The listing builds one solid part. Answer for the finished solid, in the listing's coordinates (mm). Coordinates: 2 decimals unless noted, no trailing zeros. Order: outer loops, then holes, each group sorted by start corner. A loop starts at its lowest first (then second) coordinate and runs counter-clockwise, first axis right, second up. Notation, with made-up numbers: (-34.75, 11.25) - (-27.75, 11.25) arc R7 ccw to (-27.75, 23.25) - close; hole circle Ø4 at (-7.5, -21.75). An arc over 180 degrees is marked (long way). Use one line per item in the form item = value. Start each with the question number.
Item 1: Section B-B, the plane x = -55 is taken. Write down the section's boundary in (y, z) (3 decimals).
Item 2: Consider line 1 along X through (y, z) = (2, -5); line 2 along X through (y, z) = (1.15, -7.5); line 3 along Z through (x, y) = (-3.5, 2.75). Determine where each line is inside the solid, lowest interval first. Write a range as [from, to].
Item 3: Section C-C, the plane y = 2.6 is taken. Write down the section's boundary in (x, z), and give its area (3 significant figures).
Item 4: Each of these flat-tipped pins is pushed along its axis until it touches: pin 1 Ø6.5 at (x, z) = (-5, -5) entering from +Y (3 decimals); pin 2 Ø2.5 at (x, z) = (-55, -17.82) entering from -Y. Where does it stop, or does it pass through?
Item 5: Section A-A, the plane z = -5 is taken. Write down the section's boundary in (x, y) (3 decimals).
from build123d import *

# Parameters (mm, degrees)
SKETCH1_W                 = 60
SKETCH1_H                 = 25
BOSS_EXTRUDE1_DEPTH       = 3.175
M5_CLEARANCE_HOLE2_D      = 5.5
M5_CLEARANCE_HOLE2_DEPTH  = 15
M5_CLEARANCE_HOLE2_TIP    = 1.652366702
M5X0_8_TAPPED_HOLE2_D     = 4.2
M5X0_8_TAPPED_HOLE2_DEPTH = 15
M5X0_8_TAPPED_HOLE2_TIP   = 1.2618073


with BuildPart() as part:
    # Sketch1 → Boss-Extrude1 (new body)
    with BuildSketch(Plane(origin=(0, 0, 0), x_dir=(1, 0, 0), z_dir=(0, 1, 0))):
        with Locations((-30, 12.5)):
            Rectangle(SKETCH1_W, SKETCH1_H)
    extrude(amount=BOSS_EXTRUDE1_DEPTH)

    # M5 Clearance Hole2
    with Locations(Plane(origin=(-55, 3.175, -5), x_dir=(0, 0, 1), z_dir=(0, 1, 0))):
        with Locations((0, 0), (0, 50)):
            Hole(M5_CLEARANCE_HOLE2_D / 2, depth=M5_CLEARANCE_HOLE2_DEPTH)
            with Locations((0, 0, -(M5_CLEARANCE_HOLE2_DEPTH + M5_CLEARANCE_HOLE2_TIP / 2))):  # 118° drill point
                Cone(0, M5_CLEARANCE_HOLE2_D / 2, M5_CLEARANCE_HOLE2_TIP, mode=Mode.SUBTRACT)

    # M5x0.8 Tapped Hole2
    with Locations(Plane(origin=(-55, 3.175, -17.8156), x_dir=(0, 0, 1), z_dir=(0, 1, 0))):
        with Locations((0, 0), (0, 50)):
            Hole(M5X0_8_TAPPED_HOLE2_D / 2, depth=M5X0_8_TAPPED_HOLE2_DEPTH)
            with Locations((0, 0, -(M5X0_8_TAPPED_HOLE2_DEPTH + M5X0_8_TAPPED_HOLE2_TIP / 2))):  # 118° drill point
                Cone(0, M5X0_8_TAPPED_HOLE2_D / 2, M5X0_8_TAPPED_HOLE2_TIP, mode=Mode.SUBTRACT)


solid = part.part
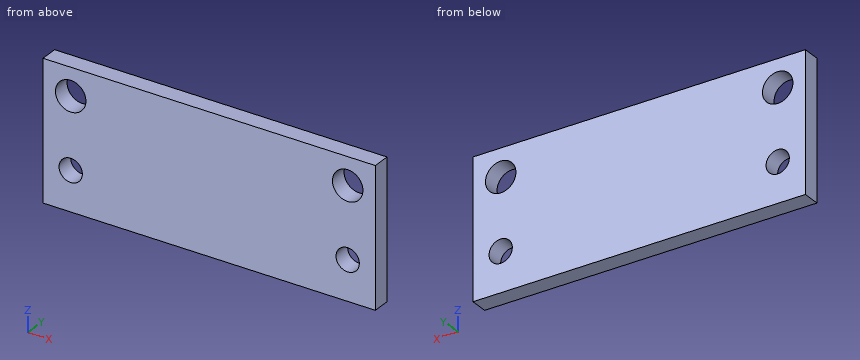
Response:
q1.outline = (0, -25) - (3.175, -25) - (3.175, -19.916) - (0, -19.916) - close; (0, -15.716) - (3.175, -15.716) - (3.175, -7.75) - (0, -7.75) - close; (0, -2.25) - (3.175, -2.25) - (3.175, 0) - (0, 0) - close
q2.line_1 = [-60, -57.75], [-52.25, -7.75], [-2.25, 0]
q2.line_2 = [-60, -56.15], [-53.85, -6.15], [-3.85, 0]
q2.line_3 = [-25, -19.29], [-16.35, -7.3], [-2.7, 0]
q3.outline = (-60, -25) - (0, -25) - (0, 0) - (-60, 0) - close; hole circle Ø5.5 at (-55, -5); hole circle Ø4.2 at (-55, -17.82); hole circle Ø5.5 at (-5, -5); hole circle Ø4.2 at (-5, -17.82)
q3.area = 1,420 mm2
q4.pin_1 = 3.175
q4.pin_2 = through
q5.outline = (-60, 0) - (-57.75, 0) - (-57.75, 3.175) - (-60, 3.175) - close; (-52.25, 0) - (-7.75, 0) - (-7.75, 3.175) - (-52.25, 3.175) - close; (-2.25, 0) - (0, 0) - (0, 3.175) - (-2.25, 3.175) - close
